Model file for the job. Use its own axes, mm. A direction names the side the tool comes from. Give positions to 0.01 mm unless a question says otherwise; leave off trailing zeros. Write each loop counter-clockwise with the first axis right and the second up, starting at its lowest first coordinate (ties: lowest second). Pieces come first, ordered by that corner, then holes. Notation, with made-up numbers: (79.25, 39.5) - (108.25, 39.5) arc R29 cw to (108.25, 77.5) - close; hole circle Ø7 at (86.25, 77.25). An arc over 180 degrees is marked (long way). Use CSV: the item, a comma, the result in double quotes.
from build123d import *

# Parameters (mm, degrees)
SKETCH_1_R               = 20
EXTRUDE_1_DEPTH          = 2
SKETCH_2_R               = 3.5
CUT_EXTRUDE_1_DEPTH      = 2
SKETCH_3_R               = 1.05
CUT_EXTRUDE_2_DEPTH      = 2
EXTRUDE_START            = 1
SKETCH_5_R               = 20
SKETCH_5_R_2             = 8.25
EXTRUDE_3_DEPTH          = 1
EXTRUDE_4_DEPTH          = 1
SKETCH_9_R               = 10.2
SKETCH_9_R_2             = 7
CUT_EXTRUDE_3_DEPTH      = 1.6
EXTRUDE_START_2          = 1.6
EXTRUDE_5_DEPTH          = 1.6
PATTERN_CIRCULAR_2_COUNT = 2
PATTERN_CIRCULAR_2_ANGLE = 180
SKETCH_13_R              = 2.75
CUT_EXTRUDE_4_DEPTH      = 1.6
FILLET_1_R               = 1.5
SKETCH_14_R              = 2.15
CUT_EXTRUDE_5_DEPTH      = 10
SKETCH_15_W              = 3
SKETCH_15_H              = 5
CUT_EXTRUDE_6_DEPTH      = 10
CHAMFER_1_SIZE           = 1


# Some blends are built 0.0001 mm under size
with BuildPart() as part:
    # 草图1 → 凸台-拉伸1 (new body)
    with BuildSketch(Plane.XY):
        Circle(SKETCH_1_R)
    extrude(amount=EXTRUDE_1_DEPTH)

    # 草图2 → 切除-拉伸1 (cut)
    with BuildSketch(Plane.XY.offset(2)):
        Circle(SKETCH_2_R)
    extrude(amount=-CUT_EXTRUDE_1_DEPTH, mode=Mode.SUBTRACT)

    # 草图3 → 切除-拉伸2 (cut)
    with BuildSketch(Plane.XY.offset(2)):
        with Locations((-5.5, 0)):
            Circle(SKETCH_3_R)
        with Locations((5.5, 0)):
            Circle(SKETCH_3_R)
    extrude(amount=-CUT_EXTRUDE_2_DEPTH, mode=Mode.SUBTRACT)

    # 草图5 → 凸台-拉伸3 (add)
    with BuildSketch(Plane(origin=(0, 0, 0), x_dir=(-1, 0, 0), z_dir=(0, 0, -1)).offset(EXTRUDE_START)):
        Circle(SKETCH_5_R)
        Circle(SKETCH_5_R_2, mode=Mode.SUBTRACT)
    extrude(amount=-EXTRUDE_3_DEPTH)

    # 草图8 → 凸台-拉伸4 (add)
    with BuildSketch(Plane(origin=(0, 0, 0), x_dir=(-1, 0, 0), z_dir=(0, 0, -1))):
        with BuildLine():
            ThreePointArc((3.176136364, 1.470427761), (6.265465545, 2.641318326), (8.25, 0))
            ThreePointArc((8.25, 0), (0, 8.25), (-8.25, 0))
            ThreePointArc((-8.25, 0), (-6.265465545, 2.641318326), (-3.176136364, 1.470427761))
            ThreePointArc((-3.176136364, 1.470427761), (0, 3.5), (3.176136364, 1.470427761))
        make_face()
        with BuildLine():
            ThreePointArc((-8.25, 0), (0, -8.25), (8.25, 0))
            ThreePointArc((8.25, 0), (6.265465545, -2.641318326), (3.176136364, -1.470427761))
            ThreePointArc((3.176136364, -1.470427761), (0, -3.5), (-3.176136364, -1.470427761))
            ThreePointArc((-3.176136364, -1.470427761), (-6.265465545, -2.641318326), (-8.25, 0))
        make_face()
    extrude(amount=EXTRUDE_4_DEPTH)

    # 草图9 → 切除-拉伸3 (cut)
    with BuildSketch(Plane(origin=(0, 0, -1), x_dir=(-1, 0, 0), z_dir=(0, 0, -1))):
        Circle(SKETCH_9_R)
        Circle(SKETCH_9_R_2, mode=Mode.SUBTRACT)
    extrude(amount=-CUT_EXTRUDE_3_DEPTH, mode=Mode.SUBTRACT)

    # 草图12 → 凸台-拉伸5 (add)
    with BuildSketch(Plane(origin=(0, 0, 0.6), x_dir=(-1, 0, 0), z_dir=(0, 0, -1)).offset(EXTRUDE_START_2)):
        with BuildLine():
            Line((6.344154509, 2.958327832), (9.244339428, 4.31070627))
            ThreePointArc((9.244339428, 4.31070627), (10.2, 0), (9.244339428, -4.31070627))
            Line((9.244339428, -4.31070627), (6.344154509, -2.958327832))
            ThreePointArc((6.344154509, -2.958327832), (7, 0), (6.344154509, 2.958327832))
        make_face()
    extrude_5 = extrude(amount=-EXTRUDE_5_DEPTH)

    # 阵列(圆周)2: 凸台-拉伸5 ×2 about axis
    pattern_circular_2_axis = Axis((0, 0, 0), (0, 0, 1))
    for i in range(1, PATTERN_CIRCULAR_2_COUNT):
        add(extrude_5.rotate(pattern_circular_2_axis, i * PATTERN_CIRCULAR_2_ANGLE / (PATTERN_CIRCULAR_2_COUNT - 1)))

    # 草图13 → 切除-拉伸4 (cut)
    with BuildSketch(Plane(origin=(0, 0, 0), x_dir=(-1, 0, 0), z_dir=(0, 0, -1))):
        with Locations((5.5, 0)):
            Circle(SKETCH_13_R)
        with Locations((-5.5, 0)):
            Circle(SKETCH_13_R)
    extrude(amount=CUT_EXTRUDE_4_DEPTH, mode=Mode.SUBTRACT)

    # 圆角1
    # the kernel refuses this fillet: 1.5 mm, written as the material it adds along each edge
    with BuildSketch(Plane(origin=(9.244339428, 4.31070627, -1), x_dir=(-0.49945721190303094, 0.8663385559225971, 0), z_dir=(0, 0, 1)), Plane(origin=(-9.244339428, -4.31070627, -1), x_dir=(0.49945721190302483, -0.8663385559226006, 0), z_dir=(0, 0, 1))) as fillet_1_piece_1:
        with BuildLine():
            CenterArc((1.635444705, 1.494373677), FILLET_1_R, 175.035904079, 99.928191842)
            Line((0.141071027, 1.624170876), (0, 0))
            ThreePointArc((0, 0), (0.882620952, -0.038258995), (1.765241903, 0))
        make_face()
    extrude(amount=1.6)
    with BuildSketch(Plane(origin=(9.244339428, -4.31070627, -1), x_dir=(-0.49945721190301884, -0.8663385559226039, 0), z_dir=(0, 0, 1)), Plane(origin=(-9.244339428, 4.31070627, -1), x_dir=(0.4994572119030254, 0.8663385559226003, 0), z_dir=(0, 0, 1))) as fillet_1_piece_2:
        with BuildLine():
            CenterArc((1.635444705, -1.494373677), FILLET_1_R, 85.035904079, 99.928191842)
            Line((0.141071027, -1.624170876), (0, 0))
            ThreePointArc((0, 0), (0.882620952, 0.038258995), (1.765241903, 0))
        make_face()
    extrude(amount=1.6)
    with BuildSketch(Plane(origin=(-6.344154509, 2.958327832, -1), x_dir=(-0.9063077870366493, 0.42261826174070083, 0), z_dir=(0, 0, 1)), Plane(origin=(6.344154509, -2.958327832, -1), x_dir=(0.9063077870366523, -0.4226182617406945, 0), z_dir=(0, 0, 1))) as fillet_1_piece_3:
        with BuildLine():
            CenterArc((1.366600265, -1.5), FILLET_1_R, 90, 79.835751378)
            ThreePointArc((-0.109858605, -1.235294118), (-0.027518743, -0.620084766), (0, 0))
            Line((0, 0), (1.366600265, 0))
        make_face()
    extrude(amount=1.6)
    with BuildSketch(Plane(origin=(-6.344154509, -2.958327832, -1), x_dir=(-0.9063077870366493, -0.4226182617407009, 0), z_dir=(0, 0, 1)), Plane(origin=(6.344154509, 2.958327832, -1), x_dir=(0.9063077870366462, 0.42261826174070743, 0), z_dir=(0, 0, 1))) as fillet_1_piece_4:
        with BuildLine():
            CenterArc((1.366600265, 1.5), FILLET_1_R, 190.164248622, 79.835751378)
            ThreePointArc((-0.109858605, 1.235294118), (-0.027518743, 0.620084766), (0, 0))
            Line((0, 0), (1.366600265, 0))
        make_face()
    extrude(amount=1.6)

    # 草图14 → 切除-拉伸5 (cut)
    with BuildSketch(Plane(origin=(0, 0, -1), x_dir=(-1, 0, 0), z_dir=(0, 0, -1))):
        with Locations((9.899494937, -9.899494937)):
            Circle(SKETCH_14_R)
        with Locations((-9.899494937, -9.899494937)):
            Circle(SKETCH_14_R)
        with Locations((-9.899494937, 9.899494937)):
            Circle(SKETCH_14_R)
        with Locations((9.899494937, 9.899494937)):
            Circle(SKETCH_14_R)
    extrude(amount=-CUT_EXTRUDE_5_DEPTH, mode=Mode.SUBTRACT)

    # 草图15 → 切除-拉伸6 (cut)
    with BuildSketch(Plane.XY.offset(2)):
        with Locations((-14, 0)):
            Rectangle(SKETCH_15_W, SKETCH_15_H)
        with Locations((14, 0)):
            Rectangle(SKETCH_15_W, SKETCH_15_H)
    extrude(amount=-CUT_EXTRUDE_6_DEPTH, mode=Mode.SUBTRACT)

    # 倒角1
    chamfer_1_edges = [part.edges().sort_by_distance(p)[0] for p in [
        (20, 0, -1),
    ]]
    chamfer(chamfer_1_edges, length=CHAMFER_1_SIZE - 0.0001)  # a hair under: the kernel refuses the full size


solid = part.part
(1) Wall check: probe 1 along X at (y, z) = (0.5, 1.7); probe 2 along Y at (x, z) = (10.5, 0.1); probe 3 along X at (y, z) = (-2, 0.15). Give the ranges that are in metal, low to high. Write a range as [from, to].
Checked values:
probe 1,"x = [-19.99, -15.5], [-12.5, -6.42], [-4.58, -3.46], [3.46, 4.58], [6.42, 12.5], [15.5, 19.99]"
probe 2,"y = [-17.02, -11.96], [-7.84, 7.84], [11.96, 17.02]"
probe 3,"x = [-19.9, -15.5], [-12.5, -2.87], [2.87, 12.5], [15.5, 19.9]"
(2) Saw through at B-B, the plane x = 0. List the corners of the cut face in (y, z).
Checked values:
outline,"(-20, 0) - (-19, -1) - (-10.2, -1) - (-10.2, 0.6) - (-7, 0.6) - (-7, -1) - (-3.5, -1) - (-3.5, 2) - (-20, 2) - close; (3.5, -1) - (7, -1) - (7, 0.6) - (10.2, 0.6) - (10.2, -1) - (19, -1) - (20, 0) - (20, 2) - (3.5, 2) - close"
(3) 3-axis set-ups, long thin cutter, end or side, ignore diameter. For faces 4 (the face through (-14, 2.5, 1)), 5 (the face through (6.55, 3.45, -0.21)): which of +Z, -Z, +X, -X, +Y, -Y reach the whole face in a straight line?
Checked values:
face 4,"+Z, -Z"
face 5,"-Z"
(4) Saw through at A-A, the plane y = 0. Count the separate pieces of the cut face and the enclosed holes in it, then the cut area to 3 significant figures.
Checked values:
separate pieces,"6"
enclosed holes,"0"
area,"62.1 mm^2"
(5) Pull direction Y, two halves, no side cores. Call faces 1 (the face through (-6.58, 3.44, -0.21)), 2 (the face through (4.45, 0.05, 1.01)), 3 (the face through (4, 0, 2)): released by +Y, released by -Y, zero draft, split by the parting line, or undercut.
Checked values:
face 1,"undercut"
face 2,"undercut"
face 3,"zero draft"
(6) Flat gauge pins, fed straight in: P1, Ø0.9, axis at x = -14, z = 0, coming from the -Y side; P2, Ø6.5, axis at x = 0, y = 0, coming from the +Z side; P3, Ø1.9, axis at x = -5, y = -1.5, coming from the -Z side; P4, Ø0.9, axis at y = 1, z = 0, coming from the -X side. Where does each tip first touch, or does it go through?
Checked values:
P1,"stops at y = -14.71"
P2,"passes through"
P3,"stops at z = 0"
P4,"stops at x = -19.99"
